from build123d import *

# Parameters (mm, degrees)
SKETCH1_W           = 25.4
SKETCH1_H           = 25.4
SKETCH1_W_2         = 22.225
SKETCH1_H_2         = 22.225
BOSS_EXTRUDE1_DEPTH = 812.8
SKETCH3_R           = 2.54
CUT_EXTRUDE2_DEPTH  = 814.593362805
CUT_EXTRUDE3_REACH  = 815.593
SKETCH4_R           = 2.54
CUT_EXTRUDE4_REACH  = 815.593
SKETCH5_R           = 2.54


with BuildPart() as part:
    # Sketch1 → Boss-Extrude1 (new body)
    with BuildSketch(Plane.XY):
        with Locations((12.7, 12.7)):
            Rectangle(SKETCH1_W, SKETCH1_H)
        with Locations((12.7, 12.7)):
            Rectangle(SKETCH1_W_2, SKETCH1_H_2, mode=Mode.SUBTRACT)
    extrude(amount=BOSS_EXTRUDE1_DEPTH)

    # Sketch3 → Cut-Extrude2 (cut, through all)
    with BuildSketch(Plane(origin=(0, 25.4, 0), x_dir=(1, 0, 0), z_dir=(0, 1, 0))):
        with Locations(Location((12.7, -12.7, 0), (0, 0, 270))):
            Circle(SKETCH3_R)
        with Locations(Location((12.7, -38.1, 0), (0, 0, 270))):
            Circle(SKETCH3_R)
        with Locations(Location((12.7, -774.7, 0), (0, 0, 90))):
            Circle(SKETCH3_R)
        with Locations(Location((12.7, -800.1, 0), (0, 0, 90))):
            Circle(SKETCH3_R)
        with Locations(Location((6.35, -698.5, 0), (0, 0, 270))):
            Circle(SKETCH3_R)
        with Locations(Location((6.35, -673.1, 0), (0, 0, 270))):
            Circle(SKETCH3_R)
    extrude(amount=-CUT_EXTRUDE2_DEPTH, mode=Mode.SUBTRACT)

    # Sketch4 → Cut-Extrude3 (cut, up to next)
    with BuildSketch(Plane(origin=(25.4, 0, 0), x_dir=(0, 0, -1), z_dir=(1, 0, 0)), mode=Mode.PRIVATE) as cut_extrude3_sk1:
        with Locations((-6.35, 12.7)):
            Circle(SKETCH4_R)
    cut_extrude3_tool1 = extrude(cut_extrude3_sk1.sketch, amount=-CUT_EXTRUDE3_REACH, mode=Mode.PRIVATE) & part.part
    # Sketch4 → Cut-Extrude3 (cut, up to next)
    with BuildSketch(Plane(origin=(25.4, 0, 0), x_dir=(0, 0, -1), z_dir=(1, 0, 0)), mode=Mode.PRIVATE) as cut_extrude3_sk2:
        with Locations((-31.75, 12.7)):
            Circle(SKETCH4_R)
    cut_extrude3_tool2 = extrude(cut_extrude3_sk2.sketch, amount=-CUT_EXTRUDE3_REACH, mode=Mode.PRIVATE) & part.part
    add(cut_extrude3_tool1.solids().sort_by_distance((25.4, 12.7, 6.35))[0], mode=Mode.SUBTRACT)
    add(cut_extrude3_tool2.solids().sort_by_distance((25.4, 12.7, 31.75))[0], mode=Mode.SUBTRACT)

    # Sketch5 → Cut-Extrude4 (cut, up to next)
    with BuildSketch(Plane.ZY, mode=Mode.PRIVATE) as cut_extrude4_sk1:
        with Locations((39.6875, 12.7)):
            Circle(SKETCH5_R)
    cut_extrude4_tool1 = extrude(cut_extrude4_sk1.sketch, amount=-CUT_EXTRUDE4_REACH, mode=Mode.PRIVATE) & part.part
    # Sketch5 → Cut-Extrude4 (cut, up to next)
    with BuildSketch(Plane.ZY, mode=Mode.PRIVATE) as cut_extrude4_sk2:
        with Locations((730.25, 12.7)):
            Circle(SKETCH5_R)
    cut_extrude4_tool2 = extrude(cut_extrude4_sk2.sketch, amount=-CUT_EXTRUDE4_REACH, mode=Mode.PRIVATE) & part.part
    # Sketch5 → Cut-Extrude4 (cut, up to next)
    with BuildSketch(Plane.ZY, mode=Mode.PRIVATE) as cut_extrude4_sk3:
        with Locations((755.65, 12.7)):
            Circle(SKETCH5_R)
    cut_extrude4_tool3 = extrude(cut_extrude4_sk3.sketch, amount=-CUT_EXTRUDE4_REACH, mode=Mode.PRIVATE) & part.part
    add(cut_extrude4_tool1.solids().sort_by_distance((0, 12.7, 39.6875))[0], mode=Mode.SUBTRACT)
    add(cut_extrude4_tool2.solids().sort_by_distance((0, 12.7, 730.25))[0], mode=Mode.SUBTRACT)
    add(cut_extrude4_tool3.solids().sort_by_distance((0, 12.7, 755.65))[0], mode=Mode.SUBTRACT)


solid = part.part
Source: CAD feature listing. Evaluate the final solid. Frame: model axes, mm. A direction names the side the tool comes from. Give positions to 0.01 mm unless a question says otherwise; leave off trailing zeros. Write each loop counter-clockwise with the first axis right and the second up, starting at its lowest first coordinate (ties: lowest second). Pieces come first, ordered by that corner, then holes. Notation, with made-up numbers: M 78.5,-29.5 L 132.5,-29.5 A15 ccw 132.5,-17.5 Z; hole C 4,56 d5. An arc over 180 degrees is marked long. Answer as a JSON object with one key per item and string values.
Q1. Contact query for flat-ended pins moving along their axis: P1, Ø3, axis at x = 6.35, z = 673.1, coming from the +Y side; P2, Ø3, axis at y = 12.7, z = 730.25, coming from the -X side. Output: stop coordinate, or through.
Geometry check:
{"P1": "passes through", "P2": "stops at x = 23.81"}
Q2. Cut plane A-A, the plane z = 686. Return the cut outline in (x, y).
Geometry check:
{"outline": "M 0,0 L 25.4,0 L 25.4,25.4 L 0,25.4 Z; hole M 1.59,1.59 L 23.81,1.59 L 23.81,23.81 L 1.59,23.81 Z"}
Q3. Cut plane B-B, the plane y = 5.5. Return the cut outline in (x, z), then the cut area to 3 significant figures.
Geometry check:
{"outline": "M 0,0 L 1.59,0 L 1.59,812.8 L 0,812.8 Z; M 23.81,0 L 25.4,0 L 25.4,812.8 L 23.81,812.8 Z", "area": "2,580 mm^2"}
Q4. Access query for faces 1 (the face through (13, 1.587, 401)), 2 (the face through (25.4, 13, 401)). Directions: +Z, -Z, +X, -X, +Y, -Y. A direction counts if a zero-diameter tool reaches every point of the face in a straight line with its end or side. Return the directions, or none.
Geometry check:
{"face 1": "+Z, -Z", "face 2": "+Z, -Z, +X, +Y, -Y"}
Q5. Ray query, line 1 along X through (y, z) = (7.5, 727); line 2 along X through (y, z) = (0.5, 12.7). Return the intervals inside material, ascending.
Geometry check:
{"line 1": "x = 0 to 1.59, 23.81 to 25.4", "line 2": "x = 0 to 10.16, 15.24 to 25.4"}
